Work out the finished part from the listing and answer in its coordinate system (mm). A direction names the side the tool comes from. Coordinates: 2 decimals unless noted, no trailing zeros. Write each loop counter-clockwise with the first axis right and the second up, starting at its lowest first coordinate (ties: lowest second). Pieces come first, ordered by that corner, then holes. Notation, with made-up numbers: (25, 6.5) - (76, 6.5) arc R29 cw to (76, 31.5) - close; hole circle Ø10 at (37.5, 29). An arc over 180 degrees is marked (long way). Answer as a JSON object with one key per item and string values. Group by question number.
from build123d import *

# Parameters (mm, degrees)
F0_R     = 6
F1_DEPTH = 10
F2_R     = 4.25
F3_DEPTH = 10
F4_W     = 50
F4_H     = 8
F5_DEPTH = 10


with BuildPart() as f1:
    # F0 (on Top) → F1 (new body)
    with BuildSketch(Plane.XY):
        with Locations((-33.975307, 0)):
            Circle(F0_R)
    extrude(amount=F1_DEPTH)

    # F2 (on face) → F3 (cut)
    with BuildSketch(Plane.XY.offset(10)):
        with Locations((-33.975307, 0)):
            Circle(F2_R)
    extrude(amount=-F3_DEPTH, mode=Mode.SUBTRACT)

    # F4 (on face) → F5 (join)
    with BuildSketch(Plane(origin=(0, 0, 0), x_dir=(1, 0, 0), z_dir=(0, 0, -1))):
        with Locations((-4.503171, 0)):
            Rectangle(F4_W, F4_H)
    extrude(amount=-F5_DEPTH)

    # F6: F1 across face


with BuildPart() as f1_1:
    add(f1.part)
    add(f1.part.mirror(Plane(origin=(20.496829, 0, 5), x_dir=(0, 1, 0), z_dir=(1, 0, 0))))


solid = f1_1.part
Q1. Flat-ended cylindrical pins translate along their axes: pin 1 Ø5 at (x, z) = (36, 6) entering from -Y; pin 2 Ø1 at (y, z) = (2, 2) entering from -X. Find the tip coordinate at first contact, or state that the pin passes through.
Q2. For a pull along X with two mould halves and no side action, classify faces 3 (the face through (21, 0, 0)), 4 (the face through (80.966, 0.203, 4.93)), 5 (the face through (21, 4, 5)) as +X half, -X half, draft (parallel to the pull), parting line (faces both ways), or undercut.
Q3. Consider L1, parallel to X at y = -2, z = 0.75; L2, parallel to X at y = -0.75, z = 7.5; L3, parallel to Y at x = 65.5, z = 3. Determine where each line is inside the solid, lowest interval first. Write a range as from..to.
Q4. Section B-B on z = 6.75 is taken. Determine the outline of the cut face in (x, y), plus the area to 3 significant figures.
Q5. Section A-A on y = 0 is taken. Determine the outline of the cut face in (x, z), plus the area to 3 significant figures.
Q6. A tool of negligible diameter and unlimited length cuts with its end or side. For faces 1 (the face through (21, -4, 5)), 2 (the face through (-39.97, 0.2, 4.93)), from which of +Z, -Z, +X, -X, +Y, -Y can it reach the whole face along a straight path? Write none if from no direction.
Q7. Section C-C on x = -12 is taken. Determine the outline of the cut face in (y, z), plus the area to 3 significant figures.
Numbers:
{
 "1": {"pin 1": "stops at y = -4", "pin 2": "stops at x = -39.78"},
 "2": {"face 3": "draft", "face 4": "undercut", "face 5": "undercut"},
 "3": {"L1": "x = -39.63..-37.73, -30.23..71.22, 78.72..80.63", "L2": "x = -39.93..-38.16, -29.79..70.79, 79.15..80.92", "L3": "y = -4..4"},
 "4": {"outline": "(-29.5, -4) - (70.5, -4) arc R6 ccw (long way) to (70.5, 4) - (-29.5, 4) arc R6 ccw (long way) to start; hole circle Ø8.5 at (-33.98, 0); hole circle Ø8.5 at (74.97, 0)", "area": "896 mm²"},
 "5": {"outline": "(-39.98, 0) - (-38.23, 0) - (-38.23, 10) - (-39.98, 10) - close; (-29.73, 0) - (70.72, 0) - (70.72, 10) - (-29.73, 10) - close; (79.22, 0) - (80.97, 0) - (80.97, 10) - (79.22, 10) - close", "area": "1,040 mm²"},
 "6": {"face 1": "+Z, -Z, -Y", "face 2": "+Z, -Z"},
 "7": {"outline": "(-4, 0) - (4, 0) - (4, 10) - (-4, 10) - close", "area": "80.0 mm²"}
}
